Here's how the part is built. I have some questions about the finished solid (model axes, mm). A direction names the side the tool comes from. Coordinates: 2 decimals unless noted, no trailing zeros. Loops run counter-clockwise (first coordinate to the right, second up) from the corner with the lowest first, then second, coordinate; pieces in that order, holes last.
from build123d import *

# Parameters (mm, degrees)
SKETCH3_R           = 47.4
BOSS_EXTRUDE2_DEPTH = 7.5
SKETCH4_R           = 24.15
CUT_EXTRUDE1_DEPTH  = 15
BOSS_EXTRUDE4_DEPTH = 65
SKETCH6_R           = 24.15
CUT_EXTRUDE2_DEPTH  = 5
SKETCH7_W           = 57
SKETCH7_H           = 60
CUT_EXTRUDE3_DEPTH  = 35.5
SKETCH8_R           = 27.55
CUT_EXTRUDE4_DEPTH  = 55


with BuildPart() as part:
    # Sketch3 → Boss-Extrude2 (new body)
    with BuildSketch(Plane.XY):
        Circle(SKETCH3_R)
    extrude(amount=BOSS_EXTRUDE2_DEPTH)

    # Sketch4 → Cut-Extrude1 (cut)
    with BuildSketch(Plane.XY.offset(7.5)):
        Circle(SKETCH4_R)
    extrude(amount=-CUT_EXTRUDE1_DEPTH, mode=Mode.SUBTRACT)

    # Sketch5 → Boss-Extrude4 (add)
    with BuildSketch(Plane.XY.offset(7.5)):
        Polygon((-33.5, -47.4), (33.5, -47.4), (33.5, -33.5), (33.5, 33.5), (0, 33.5), (-33.5, 33.5), (-33.5, -33.5), align=None)
    extrude(amount=BOSS_EXTRUDE4_DEPTH)

    # Sketch6 → Cut-Extrude2 (cut)
    with BuildSketch(Plane(origin=(0, 0, 7.5), x_dir=(-1, 0, 0), z_dir=(0, 0, -1))):
        Circle(SKETCH6_R)
    extrude(amount=-CUT_EXTRUDE2_DEPTH, mode=Mode.SUBTRACT)

    # Sketch7 → Cut-Extrude3 (cut)
    with BuildSketch(Plane(origin=(0, 33.5, 0), x_dir=(1, 0, 0), z_dir=(0, 1, 0))):
        with Locations((0, -37.5)):
            Rectangle(SKETCH7_W, SKETCH7_H)
    extrude(amount=-CUT_EXTRUDE3_DEPTH, mode=Mode.SUBTRACT)

    # Sketch8 → Cut-Extrude4 (cut)
    with BuildSketch(Plane(origin=(0, 0, 12.5), x_dir=(-1, 0, 0), z_dir=(0, 0, -1))):
        Circle(SKETCH8_R)
    extrude(amount=-CUT_EXTRUDE4_DEPTH, mode=Mode.SUBTRACT)


solid = part.part
Q1. We'd pull the mould along X, two halves only. Please class faces 1 (the flat face through (33.5, -8, 40)), 2 (the flat face through (0, 33.5, 69)), 3 (the flat face through (0, 3, 67.5)): pulls with the +X half, pulls with the -X half, needs draft (parallel to the pull), parting line crosses it, or undercut.
Q2. Suppose I cut it at C-C on z = 45. Write out the boundary of the cut face in (x, y), and give its area (3 significant figures).
Q3. Will these pins go through, and if not, where does the flat tip stop? P1, Ø8, axis at y = 18.5, z = 9, coming from the +X side; P2, Ø2, axis at y = 6, z = 58.5, coming from the +X side; P3, Ø10, axis at y = 37.5, z = 33, coming from the -X side.
Q4. Suppose I cut it at B-B on x = 21. Write out the boundary of the cut face in (y, z).
Q5. Suppose I cut it at D-D on x = 32. Write out the boundary of the cut face in (y, z), and give its area (3 significant figures).
Q6. For faces 4 (the flat face through (-28.5, 16, 38)), 5 (the cylindrical face through (-5.235, -23.576, 4.949)), 6 (the flat face through (-33.5, -6, 40)), 7 (the flat face through (-26, -42, 7.5)), which set-ups out of +Z, -Z, +X, -X, +Y, -Y let a thin tool reach every point of the face, with its end or its side?
Q7. Suppose I cut it at A-A on y = 0. Write out the boundary of the cut face in (x, z), and give its area (3 significant figures).
Q8. Please list where these lines run through material, in increasing order: probe 1 along Z at (x, y) = (18.5, 21); probe 2 along X at (y, z) = (0, 10); probe 3 along X at (y, z) = (0, 3.75).
Check values:
1. face 1: pulls with the +X half
1. face 2: needs draft
1. face 3: undercut
2. outline: (-33.5, -47.4) - (33.5, -47.4) - (33.5, 33.5) - (28.5, 33.5) - (28.5, -2) - (27.48, -2) arc R27.55 cw to (-27.48, -2) - (-28.5, -2) - (-28.5, 33.5) - (-33.5, 33.5) - close
2. area: 2,310 mm2
3. P1: stops at x = 45.03
3. P2: stops at x = 33.5
3. P3: stops at x = -33.5
4. outline: (-47.4, 7.5) - (-42.49, 7.5) - (-42.49, 0) - (-11.93, 0) - (-11.93, 12.5) - (-17.83, 12.5) - (-17.83, 67.5) - (33.5, 67.5) - (33.5, 72.5) - (-47.4, 72.5) - close; (11.93, 0) - (42.49, 0) - (42.49, 7.5) - (11.93, 7.5) - close
5. outline: (-47.4, 7.5) - (-34.97, 7.5) - (-34.97, 0) - (34.97, 0) - (34.97, 7.5) - (33.5, 7.5) - (33.5, 72.5) - (-47.4, 72.5) - close
5. area: 5,780 mm2
6. face 4: +Y
6. face 5: -Z
6. face 6: +Z, -X, +Y, -Y
6. face 7: -Z, -X, -Y
7. outline: (-47.4, 0) - (-24.15, 0) - (-24.15, 7.5) - (-28.5, 7.5) - (-28.5, 67.5) - (28.5, 67.5) - (28.5, 7.5) - (24.15, 7.5) - (24.15, 0) - (47.4, 0) - (47.4, 7.5) - (33.5, 7.5) - (33.5, 72.5) - (-33.5, 72.5) - (-33.5, 7.5) - (-47.4, 7.5) - close
7. area: 1,280 mm2
8. probe 1: z = 0 to 7.5, 67.5 to 72.5
8. probe 2: x = -33.5 to -28.5, 28.5 to 33.5
8. probe 3: x = -47.4 to -24.15, 24.15 to 47.4
